Geometry check sheet. Reference: the model listing, model coordinates, mm. Give positions to 0.01 mm unless a question says otherwise; leave off trailing zeros. Write each loop counter-clockwise with the first axis right and the second up, starting at its lowest first coordinate (ties: lowest second). Pieces come first, ordered by that corner, then holes.
(1) Thickness scan on line 1 along Y through (x, z) = (0, 2) (3 decimals); line 2 along Y through (x, z) = (0, 29) (3 decimals); line 3 along X through (y, z) = (-101, 26). Record the ranges inside material, lowest first.
(2) Cross-section at C-C (y = 101.6). Record the boundary of the cut face in (x, z) (3 decimals), and give its area (3 significant figures).
(3) Cross-section at A-A (x = 0). Record the boundary of the cut face in (y, z) (3 decimals), and give its area (3 significant figures).
(4) Depth check by flat-ended pin: P1, Ø10.5, axis at x = 0, y = -101.6, coming from the -Z side; P2, Ø10, axis at x = -1.5, y = 105, coming from the +Z side (3 decimals). Enter the tip coordinate at first touch or a pass-through.
(5) Cross-section at B-B (z = 37.5). Record the boundary of the cut face in (x, y) (3 decimals).
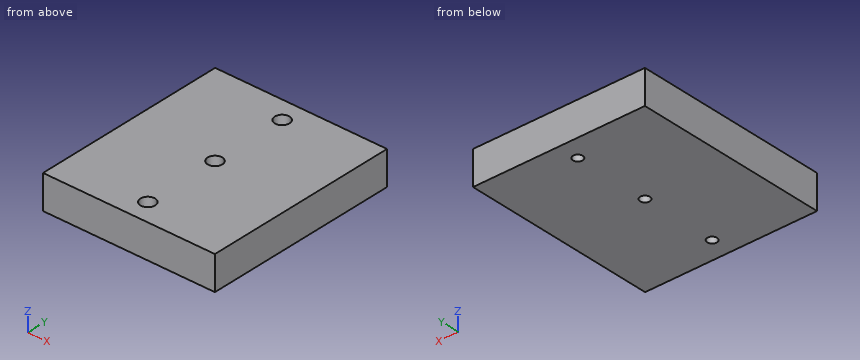
```python
from build123d import *

# Parameters (mm, degrees)
SKETCH1_W                = 228.6
SKETCH1_H                = 260.35
BOSS_EXTRUDE1_DEPTH      = 45.1104
SKETCH2_R                = 6.5151
HAAS_T_SLOT_HOLES_DEPTH  = 180.011085727
SKETCH3_R                = 9.779
HAAS_COUNTER_BORES_DEPTH = 35.5854


with BuildPart() as part:
    # Sketch1 → Boss-Extrude1 (new body)
    with BuildSketch(Plane.XY):
        Rectangle(SKETCH1_W, SKETCH1_H)
    extrude(amount=BOSS_EXTRUDE1_DEPTH)

    # Sketch2 → HAAS T-Slot Holes (cut, through all)
    with BuildSketch(Plane.XY.offset(45.1104)):
        Circle(SKETCH2_R)
        with Locations((0, 101.6)):
            Circle(SKETCH2_R)
        with Locations((0, -101.6)):
            Circle(SKETCH2_R)
    extrude(amount=-HAAS_T_SLOT_HOLES_DEPTH, mode=Mode.SUBTRACT)

    # Sketch3 → HAAS Counter Bores (cut)
    with BuildSketch(Plane.XY.offset(45.1104)):
        with Locations((0, 101.6)):
            Circle(SKETCH3_R)
        Circle(SKETCH3_R)
        with Locations((0, -101.6)):
            Circle(SKETCH3_R)
    extrude(amount=-HAAS_COUNTER_BORES_DEPTH, mode=Mode.SUBTRACT)


solid = part.part
```
Reply:
1. line 1: y = -130.175 to -108.115, -95.085 to -6.515, 6.515 to 95.085, 108.115 to 130.175
1. line 2: y = -130.175 to -111.379, -91.821 to -9.779, 9.779 to 91.821, 111.379 to 130.175
1. line 3: x = -114.3 to -9.76, 9.76 to 114.3
2. outline: (-114.3, 0) - (-6.515, 0) - (-6.515, 9.525) - (-9.779, 9.525) - (-9.779, 45.11) - (-114.3, 45.11) - close; (6.515, 0) - (114.3, 0) - (114.3, 45.11) - (9.779, 45.11) - (9.779, 9.525) - (6.515, 9.525) - close
2. area: 9,490 mm2
3. outline: (-130.175, 0) - (-108.115, 0) - (-108.115, 9.525) - (-111.379, 9.525) - (-111.379, 45.11) - (-130.175, 45.11) - close; (-95.085, 0) - (-6.515, 0) - (-6.515, 9.525) - (-9.779, 9.525) - (-9.779, 45.11) - (-91.821, 45.11) - (-91.821, 9.525) - (-95.085, 9.525) - close; (6.515, 0) - (95.085, 0) - (95.085, 9.525) - (91.821, 9.525) - (91.821, 45.11) - (9.779, 45.11) - (9.779, 9.525) - (6.515, 9.525) - close; (108.115, 0) - (130.175, 0) - (130.175, 45.11) - (111.379, 45.11) - (111.379, 9.525) - (108.115, 9.525) - close
3. area: 9,280 mm2
4. P1: passes through
4. P2: stops at z = 9.525
5. outline: (-114.3, -130.175) - (114.3, -130.175) - (114.3, 130.175) - (-114.3, 130.175) - close; hole circle Ø19.558 at (0, -101.6); hole circle Ø19.558 at (0, 0); hole circle Ø19.558 at (0, 101.6)
